```python
from build123d import *

# Parameters (mm, degrees)
SKETCH1_W            = 50
SKETCH1_H            = 44
BOSS_EXTRUDE1_DEPTH  = 2
SKETCH2_R            = 1.003593064
SKETCH2_W            = 14
SKETCH2_H            = 8
CUT_EXTRUDE1_DEPTH   = 2
LPATTERN1_COUNT      = 2
LPATTERN1_PITCH      = 41
LPATTERN1_COUNT_DIR2 = 2
LPATTERN1_PITCH_DIR2 = 36
SKETCH6_W            = 50
SKETCH6_H            = 0.998412165
CUT_EXTRUDE2_DEPTH   = 5
SKETCH7_W            = 50
SKETCH7_H            = 0.999196335
CUT_EXTRUDE3_DEPTH   = 5


with BuildPart() as part:
    # Sketch1 → Boss-Extrude1 (new body)
    with BuildSketch(Plane(origin=(0, 0, 0), x_dir=(0, 0, -1), z_dir=(1, 0, 0))):
        Rectangle(SKETCH1_W, SKETCH1_H)
    extrude(amount=BOSS_EXTRUDE1_DEPTH)

    # Sketch2 → Cut-Extrude1 (cut)
    with BuildSketch(Plane.ZY):
        with Locations((20.499792875, 18)):
            Circle(SKETCH2_R)
        with Locations((5, -13)):
            Rectangle(SKETCH2_W, SKETCH2_H)
    cut_extrude1 = extrude(amount=-CUT_EXTRUDE1_DEPTH, mode=Mode.SUBTRACT)

    # LPattern1: Cut-Extrude1 2 × 2
    with Locations(*[(0, -j * LPATTERN1_PITCH_DIR2, -i * LPATTERN1_PITCH) for i in range(LPATTERN1_COUNT) for j in range(LPATTERN1_COUNT_DIR2) if (i, j) != (0, 0)]):
        add(cut_extrude1, mode=Mode.SUBTRACT)

    # Sketch6 → Cut-Extrude2 (cut)
    with BuildSketch(Plane(origin=(2, 0, 0), x_dir=(0, 0, -1), z_dir=(1, 0, 0))):
        with Locations((0, 21.500793918)):
            Rectangle(SKETCH6_W, SKETCH6_H)
    extrude(amount=-CUT_EXTRUDE2_DEPTH, mode=Mode.SUBTRACT)

    # Sketch7 → Cut-Extrude3 (cut)
    with BuildSketch(Plane(origin=(2, 0, 0), x_dir=(0, 0, -1), z_dir=(1, 0, 0))):
        with Locations((0, -21.500401833)):
            Rectangle(SKETCH7_W, SKETCH7_H)
    extrude(amount=-CUT_EXTRUDE3_DEPTH, mode=Mode.SUBTRACT)


solid = part.part
```
Read the model definition and answer for the solid it produces. Units are mm, in the model's axes. A direction names the side the tool comes from. Give positions to 0.01 mm unless a question says otherwise; leave off trailing zeros. Loops run counter-clockwise (first coordinate to the right, second up) from the corner with the lowest first, then second, coordinate; pieces in that order, holes last.
Item 1: Find the intervals of material crossed by line 1 along Y through (x, z) = (0.4, 1); line 2 along Y through (x, z) = (0.35, 21); line 3 along Z through (x, y) = (1.25, -11), in increasing order.
Item 2: This flat-tipped pin is pushed along its axis until it touches: pin 1 Ø1.6 at (y, z) = (18, -20.5) entering from -X. Where does it stop, or does it pass through?
Item 3: The part is cut by section B-B (y = -18). Write down the section's boundary in (x, z), and give its area (3 significant figures).
Item 4: The mould has two halves that part along Z. Classify faces 3 (the flat face through (1, 0, -25)), 4 (the flat face through (1, -13, -2)), 5 (the flat face through (1, 21.002, 0)): released by +Z, released by -Z, zero draft, split by the parting line, or undercut.
Item 5: The part is cut by section A-A (z = 6.5). Write down the section's boundary in (x, y), and give its area (3 significant figures).
Item 6: The part is cut by section C-C (x = 1.3). Write down the section's boundary in (y, z), and give its area (3 significant figures).
Item 7: For faces 1 (the flat face through (1, -13, 12)), 2 (the flat face through (1, -21.001, 0)), determine the directions among +Z, -Z, +X, -X, +Y, -Y from which every point of the face is accessible in a straight line to the end or side of a thin tool.
Taken from the geometry:
1. line 1: y = -21 to -17, -9 to 21
1. line 2: y = -21 to -18.87, -17.13 to 17.13, 18.87 to 21
1. line 3: z = -25 to -2, 12 to 25
2. pin 1: passes through
3. outline: (0, -25) - (2, -25) - (2, -21.5) - (0, -21.5) - close; (0, -19.5) - (2, -19.5) - (2, 19.5) - (0, 19.5) - close; (0, 21.5) - (2, 21.5) - (2, 25) - (0, 25) - close
3. area: 92.0 mm2
4. face 3: released by -Z
4. face 4: undercut
4. face 5: zero draft
5. outline: (0, -21) - (2, -21) - (2, -17) - (0, -17) - close; (0, -9) - (2, -9) - (2, 21) - (0, 21) - close
5. area: 68.0 mm2
6. outline: (-21, -25) - (21, -25) - (21, 25) - (-21, 25) - close; hole circle Ø2.01 at (-18, -20.5); hole circle Ø2.01 at (-18, 20.5); hole (-17, -2) - (-9, -2) - (-9, 12) - (-17, 12) - close; hole circle Ø2.01 at (18, -20.5); hole circle Ø2.01 at (18, 20.5)
6. area: 1,980 mm2
7. face 1: +X, -X
7. face 2: +Z, -Z, +X, -X, -Y
